Autodesk Inventor part; units mm, degrees
sketch "Sketch2" plane through (0, 0, 0) normal (0, 0, 1) x (1, 0, 0)
  line L0 (0, 2.8582) -> (0, -2.8582) construction
  line L1 (-5.7775, 0) -> (5.7775, 0) construction
  line L2 (0, 0) -> (4, 0)
  line L3 (4, 0) -> (-4, 0)
  circle A0 centre (0, 0) radius 4
  line L4 (0, 0) -> (-2, 3.4641)
  line L5 (0, 0) -> (4, 0) construction
  line L6 (0, 0) -> (2, 3.4641)
  line L7 (0, 0) -> (4, 0) construction
  line L8 (0, 0) -> (4, 0)
  line L9 (0, 0) -> (2, -3.4641)
  line L10 (0, 0) -> (-2, -3.4641)
  line L11 (-2, 3.4641) -> (2, 3.4641)
  line L12 (2, 3.4641) -> (4, 0)
  line L13 (4, 0) -> (2, -3.4641)
  line L14 (2, -3.4641) -> (-2, -3.4641)
  line L15 (-2, -3.4641) -> (-4, 0)
  line L16 (-4, 0) -> (-2, 3.4641)
  dimension "d3" = 4
  dimension "d2" = 8
  dimension "d1" = 120
  dimension "d0" = 60
extrude "Extrusion1" add sketch "Sketch2" along normal blind 43.5 contours L6 L12 L2 | L10 L15 L3 | L3 L16 L4 | L4 L11 L6 | L2 L13 L9 | L9 L14 L10
sketch "Sketch3" plane through (0, 0, 43.5) normal (0, 0, 1) x (1, 0, 0)
  point P0 (0, 0)
  point P1 (0, 0)
hole "Hole1" at (0, 0, 43.5) direction (0, 0, -1) diameter 3.4587 depth 44
sketch "Sketch5" plane through (0, 0, 43.5) normal (0, 0, 1) x (1, 0, 0)
  line L0 (0, 0) -> (65.19, 0)
  line L1 (65.19, 0) -> (69.19, 0)
  line L2 (65.19, 0) -> (65.19, 3.464)
  line L3 (65.19, 3.464) -> (67.19, 3.464)
  line L4 (67.19, 3.464) -> (69.19, 0)
  line L5 (65.19, 3.464) -> (63.19, 3.464)
  line L6 (65.19, 0) -> (61.19, 0)
  line L7 (61.19, 0) -> (63.19, 3.464)
  line L8 (65.19, 0) -> (65.19, -3.464)
  line L9 (65.19, -3.464) -> (67.19, -3.464)
  line L10 (67.19, -3.464) -> (69.19, 0)
  line L11 (65.19, -3.464) -> (63.19, -3.464)
  line L12 (63.19, -3.464) -> (61.19, 0)
  line L13 (2, 3.4641) -> (-2, 3.4641)
  line L14 (0, 3.4641) -> (65.19, 3.464)
  line L15 (65.19, -3.464) -> (0, -3.4641)
  line L16 (-2, -3.4641) -> (2, -3.4641)
  line L17 (4, 0) -> (2, 3.4641)
  line L18 (0, 3.4641) -> (4, 0)
  line L19 (4, 0) -> (0, -3.4641)
  point P0 (2, 3.4641)
  dimension "d21" = 65.19
  dimension "d22" = 4
  dimension "d23" = 3.464
  dimension "d24" = 2
  dimension "d25" = 2
  dimension "d26" = 4
  dimension "d27" = 3.464
  dimension "d28" = 2
  dimension "d29" = 2
extrude "Extrusion2" add sketch "Sketch5" against normal blind 43.5 contours L17 L14 L7 L0 | L0 L12 L15 L19 | L7 L5 L2 L0 | L0 L8 L11 L12 | L2 L3 L4 L1 | L1 L10 L9 L8
sketch "Sketch6" plane through (0, 0, 43.5) normal (0, 0, 1) x (1, 0, 0)
  line L0 (0, 0) -> (65.19, 0)
  dimension "d32" = 65.19
hole "Hole3" at (65.19, 0, 43.5) direction (0, 0, -1) diameter 3.4587 depth 44
properties part number "Steunstuk lang" material "S235"
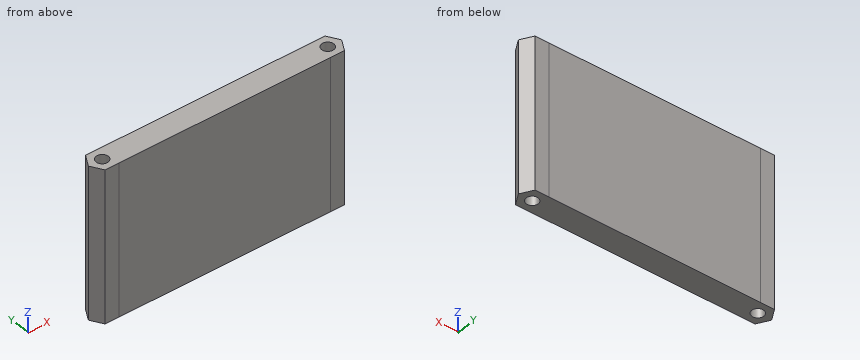
The listing builds one solid part. Answer for the finished solid, in the listing's coordinates (mm). Give positions to 0.01 mm unless a question says otherwise; leave off trailing zeros. Write each loop counter-clockwise with the first axis right and the second up, starting at its lowest first coordinate (ties: lowest second). Pieces come first, ordered by that corner, then holes.
Item 1: Section D-D, the plane y = -2.5 is taken. Write down the section's boundary in (x, z), plus the area to 3 significant figures.
Item 2: Flat-ended cylindrical pins translate along their axes: P1, Ø4, axis at y = 2.5, z = 35, coming from the -X side; P2, Ø3, axis at y = 0, z = 37.5, coming from the -X side. Find the tip coordinate at first contact, or state that the pin passes through.
Item 3: Find the intervals of material crossed by line 1 along X through (y, z) = (0, 15.5); line 2 along Y through (x, z) = (65.19, 14.5); line 3 along X through (y, z) = (-1, 29.5), in increasing order.
Item 4: Section B-B, the plane z = 27.5 is taken. Write down the section's boundary in (x, y).
Item 5: Section A-A, the plane x = 0 is taken. Write down the section's boundary in (y, z).
Completed:
1. outline: (-2.56, 0) - (67.75, 0) - (67.75, 43.5) - (-2.56, 43.5) - close
1. area: 3,060 mm2
2. P1: stops at x = -3.71
2. P2: stops at x = -4
3. line 1: x = -4 to -1.73, 1.73 to 63.46, 66.92 to 69.19
3. line 2: y = -3.46 to -1.73, 1.73 to 3.46
3. line 3: x = -3.42 to -1.41, 1.41 to 63.78, 66.6 to 68.61
4. outline: (-4, 0) - (-2, -3.46) - (2, -3.46) - (63.19, -3.46) - (67.19, -3.46) - (69.19, 0) - (67.19, 3.46) - (63.19, 3.46) - (2, 3.46) - (-2, 3.46) - close; hole circle Ø3.46 at (0, 0); hole circle Ø3.46 at (65.19, 0)
5. outline: (-3.46, 0) - (-1.73, 0) - (-1.73, 43.5) - (-3.46, 43.5) - close; (1.73, 0) - (3.46, 0) - (3.46, 43.5) - (1.73, 43.5) - close
